Here's how the part is built. I have some questions about the finished solid (model axes, mm). A direction names the side the tool comes from. Coordinates: 2 decimals unless noted, no trailing zeros. Write each loop counter-clockwise with the first axis right and the second up, starting at its lowest first coordinate (ties: lowest second). Pieces come first, ordered by that corner, then holes. Notation, with made-up numbers: (22.5, 13.5) -> (42.5, 13.5) arc R29 cw to (42.5, 50.5) -> close; hole circle Ø8 at (32.5, 6.5). An arc over 180 degrees is marked (long way). Use a Markdown table: item, result. Add a question column.
Item 1: If I drill on line 1 along X through (y, z) = (55, 6.5); line 2 along X through (y, z) = (-17, 2), over which ranges is the centre line in solid material (lowest first)? Write a range as from..to.
Item 2: Will these pins go through, and if not, where does the flat tip stop? pin 1 Ø8 at (y, z) = (40.5, 16) entering from -X; pin 2 Ø9.5 at (y, z) = (-41.5, 7) entering from -X; pin 3 Ø9.5 at (x, z) = (66.5, 11.5) entering from +Y; pin 4 Ø12 at (x, y) = (100.5, 30) entering from +Z.
Item 3: On a 3-axis mill with a long thin cutter (end or side, diameter ignored), from which of +Z, -Z, +X, -X, +Y, -Y can I reach the whole of each face in a straight line? I mean faces 5 (the flat face through (-73.902, -43.626, 9.658)), 6 (the flat face through (87.512, -37.256, 9.658)), 7 (the flat face through (146.907, 33, 10)). Say none if no direction works.
Item 4: If we mould it in two halves opening along Y, with no side actions, what happens to faces 1 (the flat face through (86.26, 33.53, 9.66)), 2 (the flat face through (13, -1, 0)), 3 (the flat face through (13, -65.869, 9)), 4 (the flat face through (146.907, -38, 10))? For each: pulls with the +Y half, pulls with the -Y half, needs draft (parallel to the pull), parting line crosses it, or undercut.
Item 5: Imagine slicing it at A-A, the plane y = 38. Write out the boundary of the cut face in (x, z).
```python
from build123d import *

# Parameters (mm, degrees)
F0_W     = 276.225
F0_H     = 127
F1_DEPTH = 19.05
F4_DEPTH = 25.4


with BuildPart() as f1:
    # F0 (on Top) → F1 (new body)
    with BuildSketch(Plane.XY):
        with Locations((15.390978, -2.369146)):
            Rectangle(F0_W, F0_H)
    extrude(amount=F1_DEPTH)

    # F3 (on face) → F4 (cut)
    with BuildSketch(Plane.XY.offset(19.05)):
        Polygon((-26.429687, 61.530381), (-146.907181, 61.530381), (-146.907181, 5.145296), align=None)
        Polygon((-146.907181, -65.84312), (-26.429687, -65.84312), (-146.907181, -9.458034), align=None)
        Polygon((146.907181, 61.530381), (26.429687, 61.530381), (146.907181, 5.145296), align=None)
        Polygon((26.429687, -65.84312), (146.907181, -65.84312), (146.907181, -9.458034), align=None)
    extrude(amount=-F4_DEPTH, mode=Mode.SUBTRACT)


solid = f1.part
```
Ans:
| question | item | result |
|---|---|---|
| 1 | line 1 | x = -40.38..40.38, 146.91..153.5 |
| 1 | line 2 | x = -122.72..130.79, 146.91..153.5 |
| 2 | pin 1 | stops at x = -79.91 |
| 2 | pin 2 | stops at x = -88.59 |
| 2 | pin 3 | stops at y = 45 |
| 2 | pin 4 | stops at z = 19.05 |
| 3 | face 5 | +Z, -Z, -X |
| 3 | face 6 | +Z, -Z |
| 3 | face 7 | +Z, -Z, +Y |
| 4 | face 1 | pulls with the +Y half |
| 4 | face 2 | needs draft |
| 4 | face 3 | pulls with the -Y half |
| 4 | face 4 | undercut |
| 5 | outline | (-76.71, 0) -> (76.71, 0) -> (76.71, 19.05) -> (-76.71, 19.05) -> close; (146.91, 0) -> (153.5, 0) -> (153.5, 19.05) -> (146.91, 19.05) -> close |
